Here's how the part is built. I have some questions about the finished solid (model axes, mm). Face numbers are marked on the shaded views. Coordinates: 2 decimals unless noted, no trailing zeros. Write each loop counter-clockwise with the first axis right and the second up, starting at its lowest first coordinate (ties: lowest second). Pieces come first, ordered by that corner, then holes. Notation, with made-up numbers: (-17, 28.25) -> (42, 28.25) arc R18 cw to (42, 63.25) -> close; hole circle Ø2 at (87.25, -31). An arc over 180 degrees is marked (long way). Put each result on its own line as item: value.
```python
from build123d import *

# Parameters (mm, degrees)
PAD_DEPTH       = 100
POCKET_DEPTH    = 8
POCKET001_DEPTH = 8


with BuildPart() as part:
    # Sketch → Pad (new body)
    with BuildSketch(Plane.XY):
        Polygon((-79.562302, -30.221603), (-9.79176, -30.556234), (-9.624449, 19.805712), (-44.760693, 50.089813), (-79.896942, 19.805712), align=None)
    extrude(amount=PAD_DEPTH)

    # Sketch001 (on Face7 of Pad) → Pocket (cut)
    with BuildSketch(Plane.XY.offset(100)):
        Polygon((-74.055283, 19.460539), (-44.906891, 44.149063), (-15.280657, 19.460539), align=None)
    extrude(amount=-POCKET_DEPTH, mode=Mode.SUBTRACT)

    # Sketch002 (on Face5 of Pocket) → Pocket001 (cut)
    with BuildSketch(Plane.XY.offset(100)):
        Polygon((-70.148895, -29.911121), (-69.888077, -3.17746), (-50.196453, -3.307868), (-50.066044, -30.302345), align=None)
        Polygon((-40.02462, 9.86335), (-39.894211, 0), (-30.896048, 0), (-30.765642, 9.86335), align=None)
        Polygon((-28.939928, 9.732944), (-20.072174, 9.993761), (-19.811361, 0), (-28.809523, 0), align=None)
        Polygon((-39.894211, -2.134194), (-30.635239, -2.264603), (-30.635239, -11.653986), (-39.763805, -11.784394), align=None)
        Polygon((-28.939928, -2.134194), (-20.072174, -2.395011), (-20.072174, -11.914803), (-28.809523, -12.045211), align=None)
    extrude(amount=-POCKET001_DEPTH, mode=Mode.SUBTRACT)


solid = part.part
```
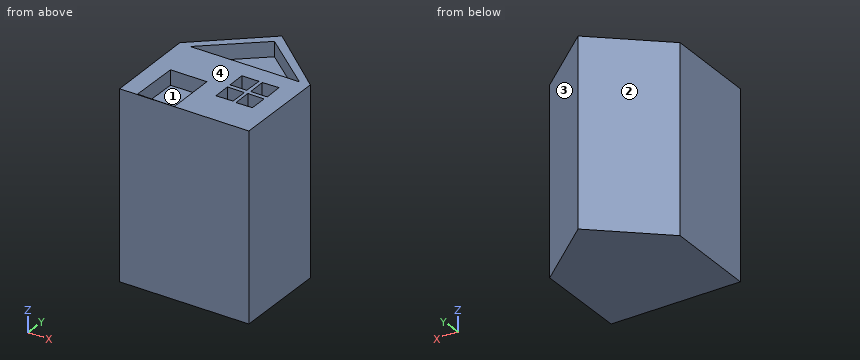
Item 1: Please list where these lines run through material, in increasing order: line 1 along Y through (x, z) = (-32, 95.5); line 2 along Z through (x, y) = (-34, -9); line 3 along Y through (x, z) = (-49.5, 12). Write a range as from..to.
Output:
line 1: y = -30.45..-11.67, -2.25..0, 9.86..19.46, 33.39..39.09
line 2: z = 0..92
line 3: y = -30.37..46
Item 2: Imagine slicing it at B-B on y = -16. Write out the boundary of the cut face in (x, z).
Output:
outline: (-79.66, 0) -> (-9.74, 0) -> (-9.74, 100) -> (-50.14, 100) -> (-50.14, 92) -> (-70.01, 92) -> (-70.01, 100) -> (-79.66, 100) -> close
Item 3: Imagine slicing it at C-C on z = 11.5. Write out the boundary of the cut face in (x, y).
Output:
outline: (-79.9, 19.81) -> (-79.56, -30.22) -> (-9.79, -30.56) -> (-9.62, 19.81) -> (-44.76, 50.09) -> close
Item 4: If we mould it in two halves opening along X, with no side actions, what happens to the marked faces 1, 2, 3 and 4? For each: released by +X, released by -X, zero draft, split by the parting line, or undercut.
Output:
face 1: undercut
face 2: released by -X
face 3: released by +X
face 4: zero draft
Item 5: For P1, Ø2, axis at x = -44, z = 46, coming from the -Y side; P2, Ø2.5, axis at x = -49, z = 96, coming from the +Y side; P3, Ø6, axis at x = -64, y = -19.5, coming from the +Z side, each with a flat end and sliding along its axis, tell me the tip position at first contact or that it passes through.
Output:
P1: stops at y = -30.4
P2: stops at y = 47.51
P3: stops at z = 92
Item 6: Imagine slicing it at A-A on x = -17.5. Write out the boundary of the cut face in (y, z).
Output:
outline: (-30.52, 0) -> (26.59, 0) -> (26.59, 100) -> (21.31, 100) -> (21.31, 92) -> (19.46, 92) -> (19.46, 100) -> (-30.52, 100) -> close
Item 7: Imagine slicing it at D-D on x = -67. Write out the boundary of the cut face in (y, z), then the cut area to 3 significant figures.
Output:
outline: (-30.28, 0) -> (30.92, 0) -> (30.92, 100) -> (25.44, 100) -> (25.44, 92) -> (19.46, 92) -> (19.46, 100) -> (-3.2, 100) -> (-3.2, 92) -> (-29.97, 92) -> (-29.97, 100) -> (-30.28, 100) -> close
area: 5,860 mm²
